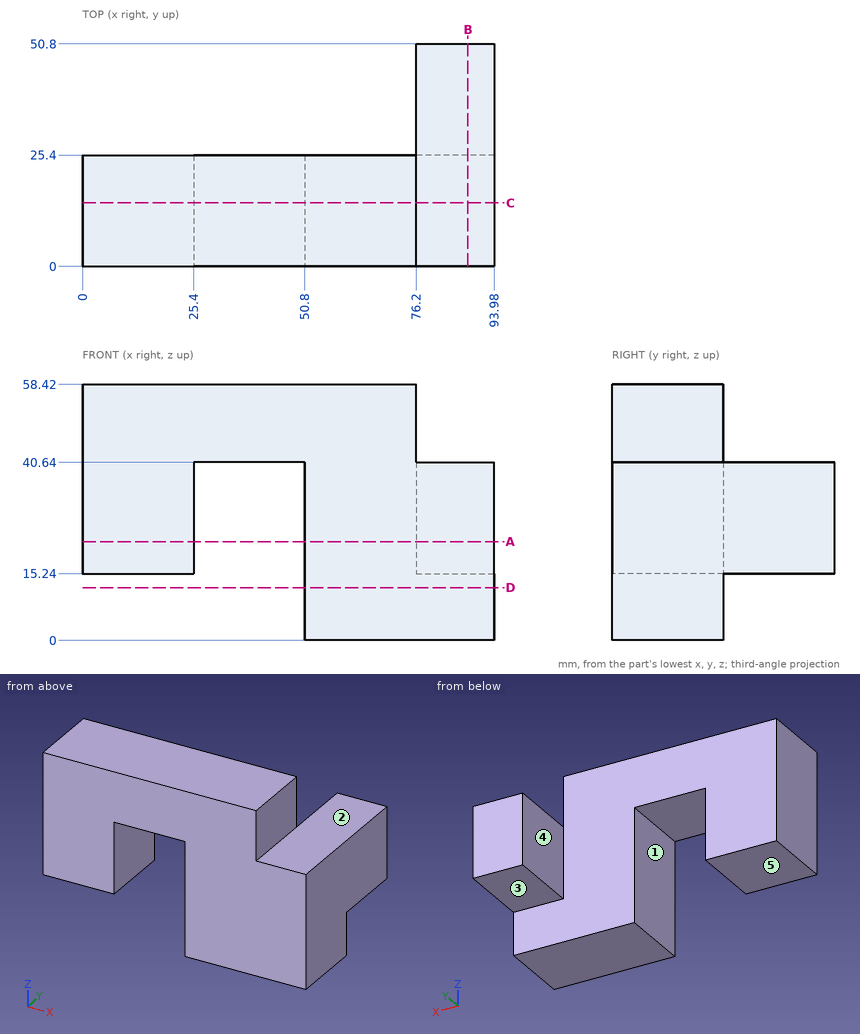
Source: three-view drawing plus pictorial views. Frame: mm from the lowest corner of the part. A direction names the side the tool comes from. Round coordinates to 2 decimals unless told otherwise and drop trailing zeros. Loops run counter-clockwise (first coordinate to the right, second up) from the corner with the lowest first, then second, coordinate; pieces in that order, holes last. Notation, with made-up numbers: (44.5, -40) - (102.5, -40) arc R19 ccw to (102.5, -17) - close; hole circle Ø4 at (9.25, 14.25). An arc over 180 degrees is marked (long way). Write each question's results on one line, items separated by ' | '. Start each with the question number.
1) Cut plane A-A on z = 22.5. Return loops of the section in (x, y).
2) Cut plane B-B on x = 88. Return loops of the section in (y, z), then the cut area to 3 significant figures.
3) Cut plane D-D on z = 12. Return loops of the section in (x, y), then the cut area to 3 significant figures.
4) First-contact query: P1, Ø12.5, axis at x = 11.5, y = 7.5, coming from the -Z side; P2, Ø1, axis at x = 79, y = 21, coming from the +Z side; P3, Ø8, axis at y = 11.5, z = 8, coming from the -X side. Flat tips, straight axial feed; report the tip coordinate or a pass-through.
5) Line query: probe 1 along Z at (x, y) = (81, 36); probe 2 along Y at (x, z) = (4, 22); probe 3 along Z at (x, y) = (77, 15.5). Output: solid intervals per line, ascending. Write a range as [from, to].
6) Cut plane C-C on y = 14.5. Return loops of the section in (x, z).
7) Access query for the marked faces 1, 2, 3, 4 and 5. Directions: +Z, -Z, +X, -X, +Y, -Y. A direction counts if a zero-diameter tool reaches every point of the face in a straight line with its end or side. Return the directions, or none.
Verdict:
1) outline: (0, 0) - (25.4, 0) - (25.4, 25.4) - (0, 25.4) - close; (50.8, 0) - (93.98, 0) - (93.98, 50.8) - (76.2, 50.8) - (76.2, 25.4) - (50.8, 25.4) - close
2) outline: (0, 0) - (25.4, 0) - (25.4, 15.24) - (50.8, 15.24) - (50.8, 40.64) - (0, 40.64) - close | area: 1,680 mm2
3) outline: (50.8, 0) - (93.98, 0) - (93.98, 25.4) - (50.8, 25.4) - close | area: 1,100 mm2
4) P1: stops at z = 15.24 | P2: stops at z = 40.64 | P3: stops at x = 50.8
5) probe 1: z = [15.24, 40.64] | probe 2: y = [0, 25.4] | probe 3: z = [0, 40.64]
6) outline: (0, 15.24) - (25.4, 15.24) - (25.4, 40.64) - (50.8, 40.64) - (50.8, 0) - (93.98, 0) - (93.98, 40.64) - (76.2, 40.64) - (76.2, 58.42) - (0, 58.42) - close
7) face 1: -Z, +Y, -Y | face 2: +Z, +X, +Y, -Y | face 3: -Z, +X, -X, +Y | face 4: +Z, -Z, -X, +Y | face 5: -Z, -X, +Y, -Y
